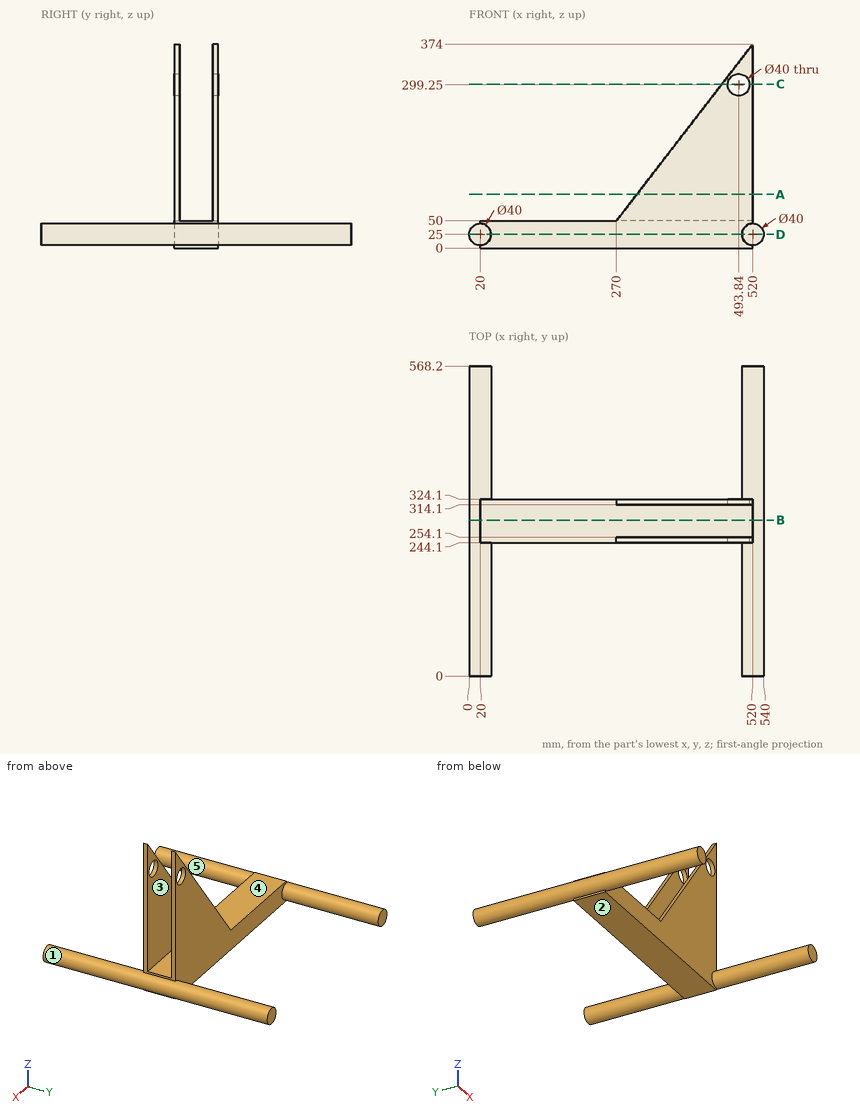
Source: three-view drawing plus pictorial views. Frame: mm from the lowest corner of the part. A direction names the side the tool comes from. Give positions to 0.01 mm unless a question says otherwise; leave off trailing zeros. Loops run counter-clockwise (first coordinate to the right, second up) from the corner with the lowest first, then second, coordinate; pieces in that order, holes last.
1) Mould query, pull axis X, two halves, no side actions, for the marked faces 4 and 5. Classes: released by +X, released by -X, zero draft, split by the parting line, or undercut.
A:
face 4: zero draft
face 5: undercut
2) Section query C-C on z = 300.5. Return the cut outline in (x, y), and give its area (3 significant figures).
A:
outline: (463.29, 244.1) - (473.88, 244.1) - (473.88, 254.1) - (463.29, 254.1) - close; (463.29, 314.1) - (473.88, 314.1) - (473.88, 324.1) - (463.29, 324.1) - close; (513.8, 244.1) - (520, 244.1) - (520, 254.1) - (513.8, 254.1) - close; (513.8, 314.1) - (520, 314.1) - (520, 324.1) - (513.8, 324.1) - close
area: 336 mm2
3) Section query A-A on z = 98.5. Return the cut outline in (x, y), and give its area (3 significant figures).
A:
outline: (307.42, 244.1) - (520, 244.1) - (520, 254.1) - (307.42, 254.1) - close; (307.42, 314.1) - (520, 314.1) - (520, 324.1) - (307.42, 324.1) - close
area: 4,250 mm2
4) Section query D-D on z = 25. Return the cut outline in (x, y).
A:
outline: (0, 0) - (40, 0) - (40, 244.1) - (500, 244.1) - (500, 0) - (540, 0) - (540, 568.2) - (500, 568.2) - (500, 324.1) - (40, 324.1) - (40, 568.2) - (0, 568.2) - close
5) Section query B-B on y = 285.5. Return the cut outline in (x, z).
A:
outline: (20, 0) - (520, 0) - (520, 5) arc R20 ccw to (520, 45) - (520, 50) - (20, 50) - (20, 45) arc R20 ccw to (20, 5) - close
6) Contact query for flat-ended pins moving along their axis: pin 1 (5.5 mm diameter, centred on y = 279.5, z = 48, fed in from -X); pin 2 (1 mm diameter, centred on x = 442.5, z = 72, fed in from -Y). Output: stop coordinate, or through.
A:
pin 1: stops at x = 20
pin 2: stops at y = 244.1
7) Reachability of the marked faces 1, 2 and 3 from +Z, -Z, +X, -X, +Y, -Y: full face, straight path, thin tool, end or side. Return the list, or none.
A:
face 1: none
face 2: -Z, +X, -X, +Y, -Y
face 3: +Z, +X, -X
8) Line query: L1, parallel to Y at x = 284.5, z = 42; L2, parallel to Z at x = 154, y = 248; L3, parallel to Z at x = 518.5, y = 101. Output: solid intervals per line, ascending.
A:
L1: y = 244.1 to 324.1
L2: z = 0 to 50
L3: z = 5.06 to 44.94
